Verification items for the finished model (mm, model axes). Face numbers are marked on the shaded views. A direction names the side the tool comes from. Coordinates: 2 decimals unless noted, no trailing zeros. Write each loop counter-clockwise with the first axis right and the second up, starting at its lowest first coordinate (ties: lowest second). Pieces come first, ordered by that corner, then holes. Notation, with made-up numbers: M 50,6 L 70,6 A18 cw 70,15 Z; hole C -18.5,46.5 d2. An arc over 180 degrees is marked long. One line per item, written item: value.
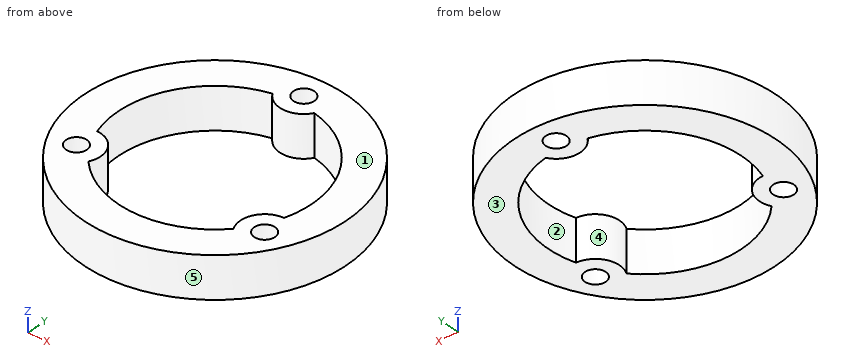
```python
from build123d import *

# Parameters (mm, degrees)
ESQUISSE1_R        = 19
ESQUISSE1_R_2      = 1.5
BOSS_EXTRU_2_DEPTH = 6


with BuildPart() as part:
    # Esquisse1 → Boss.-Extru.2 (new body)
    with BuildSketch(Plane.XY):
        Circle(ESQUISSE1_R)
        with Locations((-0.546712729, 15.490355231)):
            Circle(ESQUISSE1_R_2, mode=Mode.SUBTRACT)
        with Locations((-13.14168478, -8.218644727)):
            Circle(ESQUISSE1_R_2, mode=Mode.SUBTRACT)
        with Locations((13.688397508, -7.271710504)):
            Circle(ESQUISSE1_R_2, mode=Mode.SUBTRACT)
        with BuildLine():
            ThreePointArc((-3.468577117, 13.56351624), (-0.423261467, 11.992533082), (2.503723019, 13.774301109))
            ThreePointArc((2.503723019, 13.774301109), (11.869908833, 7.423292012), (13.480638187, -3.777882222))
            ThreePointArc((13.480638187, -3.777882222), (10.597469039, -5.629711358), (10.677033171, -9.055438293))
            ThreePointArc((10.677033171, -9.055438293), (0.493805045, -13.991288596), (-10.01206107, -9.785634018))
            ThreePointArc((-10.01206107, -9.785634018), (-10.174207571, -6.362821724), (-13.180756189, -4.718862816))
            ThreePointArc((-13.180756189, -4.718862816), (-12.363713879, 6.567996584), (-3.468577117, 13.56351624))
        make_face(mode=Mode.SUBTRACT)
    extrude(amount=BOSS_EXTRU_2_DEPTH)


solid = part.part
```
Item 1: Cross-section at D-D, the plane z = 2.3. Enter the section's corners in (x, y), and give its area (3 significant figures).
The answers:
outline: C 0,0 d38; hole C -13.14,-8.22 d3; hole M -13.18,-4.72 A3.5 cw -10.01,-9.79 A14 ccw 10.68,-9.06 A3.5 cw 13.48,-3.78 A14 ccw 2.5,13.77 A3.5 cw -3.47,13.56 A14 ccw Z; hole C -0.55,15.49 d3; hole C 13.69,-7.27 d3
area: 522 mm²
Item 2: Go/stop test with flat-tipped pins: P1, Ø8, axis at x = 4, y = -8, coming from the -Z side; P2, Ø1, axis at y = 5, z = 2, coming from the -X side. Record where each tip stops, or that it passes through.
The answers:
P1: passes through
P2: stops at x = -18.46
Item 3: Cross-section at B-B, the plane x = -7. Enter the section's corners in (y, z).
The answers:
outline: M -17.66,0 L -12.12,0 L -12.12,6 L -17.66,6 Z; M 12.12,0 L 17.66,0 L 17.66,6 L 12.12,6 Z
Item 4: Access from +Z, -Z, +X, -X, +Y, -Y to the whole of each face (thin tool, end or side, straight path). Record for the marked faces 1 and 2.
The answers:
face 1: +Z, +X, -X, +Y, -Y
face 2: +Z, -Z
Item 5: Draft check along X on the marked faces 3, 4 and 5. Enter one of: released by +X, released by -X, zero draft, split by the parting line, or undercut.
The answers:
face 3: zero draft
face 4: undercut
face 5: split by the parting line
Item 6: Scan lines: line 1 (Y direction, x = -13, z = 5.7); line 2 (X direction, y = -6.5, z = 0.9); line 3 (Y direction, x = -1.5, z = 4.45). Record each from-to range of solid material in increasing order.
The answers:
line 1: y = -13.86 to -9.71, -6.73 to -4.72, 5.2 to 13.86
line 2: x = -17.85 to -10.09, 10.27 to 12.4, 14.97 to 17.85
line 3: y = -18.94 to -13.92, 12.12 to 14.33, 16.65 to 18.94
Item 7: Cross-section at A-A, the plane y = 0. Enter the section's corners in (x, z).
The answers:
outline: M -19,0 L -14,0 L -14,6 L -19,6 Z; M 14,0 L 19,0 L 19,6 L 14,6 Z
Item 8: Cross-section at C-C, the plane x = 0. Enter the section's corners in (y, z).
The answers:
outline: M -19,0 L -14,0 L -14,6 L -19,6 Z; M 12.03,0 L 14.09,0 L 14.09,6 L 12.03,6 Z; M 16.89,0 L 19,0 L 19,6 L 16.89,6 Z
